```python
from build123d import *

# Parameters (mm, degrees)
SKETCH1_R           = 20
BOSS_EXTRUDE1_DEPTH = 1.5
SKETCH3_W           = 15
SKETCH3_H           = 10
CUT_EXTRUDE2_DEPTH  = 3


with BuildPart() as part:
    # Sketch1 → Boss-Extrude1 (new, symmetric)
    with BuildSketch(Plane(origin=(0, 0, 0), x_dir=(1, 0, 0), z_dir=(0, 1, 0))):
        with Locations(Location((0, 0, 0), (0, 0, 270))):
            Circle(SKETCH1_R)
    extrude(amount=BOSS_EXTRUDE1_DEPTH, both=True)

    # Sketch3 → Cut-Extrude2 (cut)
    with BuildSketch(Plane(origin=(0, 1.5, 0), x_dir=(1, 0, 0), z_dir=(0, 1, 0))):
        with Locations((0, 18)):
            Rectangle(SKETCH3_W, SKETCH3_H)
    cut_extrude2 = extrude(amount=-CUT_EXTRUDE2_DEPTH, mode=Mode.SUBTRACT)

    # Mirror1: Cut-Extrude2 across plane
    add(cut_extrude2.mirror(Plane.XY), mode=Mode.SUBTRACT)


solid = part.part
```
Here's how the part is built. I have some questions about the finished solid (model axes, mm). A direction names the side the tool comes from. Coordinates: 2 decimals unless noted, no trailing zeros. Order: outer loops, then holes, each group sorted by start corner. A loop starts at its lowest first (then second) coordinate and runs counter-clockwise, first axis right, second up.
Item 1: If we section it at D-D, the plane z = 10: List the corners of the cut face in (x, y) for me, then the cut area to 3 significant figures.
Response values:
outline: (-17.32, -1.5) - (17.32, -1.5) - (17.32, 1.5) - (-17.32, 1.5) - close
area: 104 mm2
Item 2: Which directions (+Z, -Z, +X, -X, +Y, -Y) give clear straight access to the entire face, cutting with the end or side of a thin tool? Please do faces 4 (the face through (-7.5, 0, 16)), 5 (the face through (0, 1.5, 0)), 6 (the face through (-7.5, 0, -16)).
Response values:
face 4: +Z, +Y, -Y
face 5: +Z, -Z, +X, -X, +Y
face 6: -Z, +Y, -Y
Item 3: I'm going to push flat-ended pins straight in: pin 1 Ø0.9 at (y, z) = (-0.5, -17) entering from +X; pin 2 Ø1 at (x, y) = (6.5, 0.5) entering from +Z; pin 3 Ø1.5 at (x, y) = (2, 0.5) entering from -Z. Where does each tip first touch, or does it pass through?
Response values:
pin 1: stops at x = 11.23
pin 2: stops at z = 13
pin 3: stops at z = -13
Item 4: If we section it at A-A, the plane z = 15: List the corners of the cut face in (x, y) for me.
Response values:
outline: (-13.23, -1.5) - (-7.5, -1.5) - (-7.5, 1.5) - (-13.23, 1.5) - close; (7.5, -1.5) - (13.23, -1.5) - (13.23, 1.5) - (7.5, 1.5) - close
Item 5: I need wall thicknesses on probe 1 along Z at (x, y) = (-2, -1); probe 2 along X at (y, z) = (1, 14); probe 3 along X at (y, z) = (0.5, 5). Which ranges of each line are inside material? Lowest first, please.
Response values:
probe 1: z = -13 to 13
probe 2: x = -14.28 to -7.5, 7.5 to 14.28
probe 3: x = -19.36 to 19.36
Item 6: If we section it at C-C, the plane x = 0.5: List the corners of the cut face in (y, z) for me.
Response values:
outline: (-1.5, -13) - (1.5, -13) - (1.5, 13) - (-1.5, 13) - close
Item 7: If we section it at B-B, the plane y = -1: List the corners of the cut face in (x, z) for me.
Response values:
outline: (-7.5, -18.54) - (-7.5, -13) - (7.5, -13) - (7.5, -18.54) arc R20 ccw to (7.5, 18.54) - (7.5, 13) - (-7.5, 13) - (-7.5, 18.54) arc R20 ccw to start
Item 8: Thinking about a two-plate mould opening in X: for faces 1 (the face through (20, 0, 0)), 2 (the face through (0, 0, 13)), 3 (the face through (-20, 0, 0)), which applies, pulls with the +X half, pulls with the -X half, needs draft (parallel to the pull), parting line crosses it, or undercut?
Response values:
face 1: pulls with the +X half
face 2: undercut
face 3: pulls with the -X half
